Geometry check sheet. Reference: the model listing, model coordinates, mm. A direction names the side the tool comes from. Give positions to 0.01 mm unless a question says otherwise; leave off trailing zeros. Loops run counter-clockwise (first coordinate to the right, second up) from the corner with the lowest first, then second, coordinate; pieces in that order, holes last. Notation, with made-up numbers: (-22, 86.25) -> (27, 86.25) arc R24 cw to (27, 107.25) -> close; hole circle Ø1 at (2, -3.75). An arc over 180 degrees is marked (long way). One line per question, with ' | ' between items.
from build123d import *

# Parameters (mm, degrees)
F0_W      = 28.2
F0_H      = 28.2
F2_DEPTH  = 2.1
F1_W      = 28.2
F1_H      = 2.1
F3_DEPTH  = 30
F4_W      = 0.5
F4_H      = 32.4
F4_W_2    = 28.2
F4_H_2    = 0.5
F5_DEPTH  = 0.5
F6_W      = 15.5
F6_H      = 36
F6_W_2    = 7
F7_DEPTH  = 2.1
F9_DEPTH  = 2.1
F10_DEPTH = 2.1
F11_W     = 33.8
F11_H     = 2.1
F12_DEPTH = 3
F13_R     = 0.325
F14_DEPTH = 35.201
F15_W     = 0.5
F15_H     = 0.5
F16_DEPTH = 25.001


with BuildPart() as f2:
    # F0 (on Top) → F2 (new body)
    with BuildSketch(Plane.XY):
        Rectangle(F0_W, F0_H)
    extrude(amount=F2_DEPTH)

    # F1 (on Top) → F3 (join)
    with BuildSketch(Plane.XY):
        Polygon((-16.2, 16.2), (-16.2, -16.2), (-14.1, -16.2), (-14.1, -14.1), (-14.1, 14.1), (-14.1, 16.2), align=None)
        with Locations((0, -15.15)):
            Rectangle(F1_W, F1_H)
        Polygon((14.1, -14.1), (14.1, -16.2), (16.2, -16.2), (16.2, 16.2), (14.1, 16.2), (14.1, 14.1), align=None)
        with Locations((0, 15.15)):
            Rectangle(F1_W, F1_H)
    extrude(amount=F3_DEPTH)

    # F4 (on face) → F5 (join)
    with BuildSketch(Plane.XY.offset(30)):
        with Locations((-15.35, 0)):
            Rectangle(F4_W, F4_H)
        with Locations((15.35, 0)):
            Rectangle(F4_W, F4_H)
        with Locations((0, 15.35)):
            Rectangle(F4_W_2, F4_H_2)
        with Locations((0, -15.35)):
            Rectangle(F4_W_2, F4_H_2)
    extrude(amount=F5_DEPTH)

    # F6 (on face) → F7 (join)
    with BuildSketch(Plane.XY.offset(30.5)):
        with Locations((-11.25, -0.8)):
            Rectangle(F6_W, F6_H)
        with Locations((4.25, -0.8)):
            Rectangle(F6_W, F6_H)
        with Locations((15.5, -0.8)):
            Rectangle(F6_W_2, F6_H)
    extrude(amount=F7_DEPTH)

    # F8 (on face) → F9 (cut, through all)
    with BuildSketch(Plane.XZ.offset(16.2)):
        with BuildLine():
            ThreePointArc((0, 17.3), (0.707107, 17.592893), (1, 18.3))
            ThreePointArc((1, 18.3), (0.707107, 19.007107), (0, 19.3))
            ThreePointArc((0, 19.3), (-1, 18.3), (0, 17.3))
        make_face()
    extrude(amount=-F9_DEPTH, mode=Mode.SUBTRACT)

    # F8 (on face) → F10 (join)
    with BuildSketch(Plane.XZ.offset(16.2)):
        Polygon((6, 17.3), (0, 17.3), (-6, 17.3), (-6, 15.2), (6, 15.2), align=None)
        Polygon((-6, 19.3), (0, 19.3), (6, 19.3), (6, 21.4), (-6, 21.4), align=None)
    extrude(amount=F10_DEPTH)

    # F11 (on face) → F12 (join)
    with BuildSketch(Plane.XY.offset(30.5)):
        Polygon((16.9, -16.7), (16.9, -18.8), (19, -18.8), (19, 17.2), (16.9, 17.2), align=None)
        with Locations((0, -17.75)):
            Rectangle(F11_W, F11_H)
        Polygon((-19, -18.8), (-16.9, -18.8), (-16.9, -16.7), (-16.9, 17.2), (-19, 17.2), align=None)
    extrude(amount=-F12_DEPTH)

    # F13 (on face) → F14 (cut, through all)
    with BuildSketch(Plane(origin=(-16.2, 0, 0), x_dir=(0, -1, 0), z_dir=(-1, 0, 0))):
        with Locations((-11.2, 26.5)):
            Circle(F13_R)
        with Locations((-8.7, 24.5)):
            Circle(F13_R)
        with Locations((-6.2, 26.5)):
            Circle(F13_R)
        with Locations((-3.7, 24.5)):
            Circle(F13_R)
        with Locations((-1.2, 26.5)):
            Circle(F13_R)
        with Locations((1.3, 24.5)):
            Circle(F13_R)
        with Locations((3.8, 26.5)):
            Circle(F13_R)
        with Locations((6.3, 24.5)):
            Circle(F13_R)
        with Locations((8.8, 26.5)):
            Circle(F13_R)
        with Locations((11.3, 24.5)):
            Circle(F13_R)
    extrude(amount=-F14_DEPTH, mode=Mode.SUBTRACT)

    # F15 (on face) → F16 (cut, through all)
    with BuildSketch(Plane.YZ.offset(6)):
        with Locations((-17.45, 17.05)):
            Rectangle(F15_W, F15_H)
        with Locations((-17.45, 19.55)):
            Rectangle(F15_W, F15_H)
    extrude(amount=-F16_DEPTH, mode=Mode.SUBTRACT)


solid = f2.part
Item 1: Release check for a two-part mould opening along Y. For faces 1 (the face through (-16.9, 0, 29)), 2 (the face through (-14.1, 0, 16)), 3 (the face through (0, -18.3, 16)) record: pulls with the +Y half, pulls with the -Y half, needs draft (parallel to the pull), parting line crosses it, or undercut.
Result:
face 1: needs draft | face 2: undercut | face 3: pulls with the -Y half
Item 2: Sectioned sample at B-B (y = -10). Record the cut outline in (x, z).
Result:
outline: (-19, 27.5) -> (-16.9, 27.5) -> (-16.9, 30.5) -> (-15.6, 30.5) -> (-15.6, 30) -> (-16.2, 30) -> (-16.2, 0) -> (16.2, 0) -> (16.2, 30) -> (15.6, 30) -> (15.6, 30.5) -> (16.9, 30.5) -> (16.9, 27.5) -> (19, 27.5) -> (19, 32.6) -> (-19, 32.6) -> close; hole (-15.1, 30) -> (-14.1, 30) -> (-14.1, 2.1) -> (14.1, 2.1) -> (14.1, 30) -> (15.1, 30) -> (15.1, 30.5) -> (-15.1, 30.5) -> close
Item 3: Sectioned sample at A-A (z = 3). Record the cut outline in (x, y), plus the area to 3 significant figures.
Result:
outline: (-16.2, -16.2) -> (16.2, -16.2) -> (16.2, 16.2) -> (-16.2, 16.2) -> close; hole (-14.1, -14.1) -> (14.1, -14.1) -> (14.1, 14.1) -> (-14.1, 14.1) -> close | area: 255 mm2
Item 4: Depth check by flat-ended pin: pin 1 Ø1.5 at (x, z) = (-5, 8) entering from -Y; pin 2 Ø12 at (x, z) = (6, 7.5) entering from +Y; pin 3 Ø0.7 at (x, y) = (0, -18) entering from -Z. Enter the tip coordinate at first touch or a pass-through.
Result:
pin 1: y = -16.2 | pin 2: y = 16.2 | pin 3: z = 15.2
Item 5: Scan lines: probe 1 along Z at (x, y) = (-15.05, 6.2) (3 decimals); probe 2 along Y at (x, z) = (-15.35, 24.5) (3 decimals); probe 3 along X at (y, z) = (0, 29). Record each from-to range of solid material in increasing order.
Result:
probe 1: 0 to 26.175, 26.825 to 30, 30.5 to 32.6 | probe 2: -16.2 to -11.625, -10.975 to -6.625, -5.975 to -1.625, -0.975 to 3.375, 4.025 to 8.375, 9.025 to 16.2 | probe 3: -19 to -16.9, -16.2 to -14.1, 14.1 to 16.2, 16.9 to 19
Item 6: Sectioned sample at C-C (z = 20.5). Record the cut outline in (x, y).
Result:
outline: (-16.2, -16.2) -> (-6, -16.2) -> (-6, -18.3) -> (6, -18.3) -> (6, -16.2) -> (16.2, -16.2) -> (16.2, 16.2) -> (-16.2, 16.2) -> close; hole (-14.1, -14.1) -> (14.1, -14.1) -> (14.1, 14.1) -> (-14.1, 14.1) -> close
Item 7: Set-up check for faces 4 (the face through (-3, -17, 27.5)), 5 (the face through (-6, -17, 20)), 6 (the face through (-0.1, 14.5, 30)): record each of +Z, -Z, +X, -X, +Y, -Y from which the full face is reachable in a straight line by a thin tool's end or side.
Result:
face 4: -Y | face 5: -Z, -X, -Y | face 6: none
